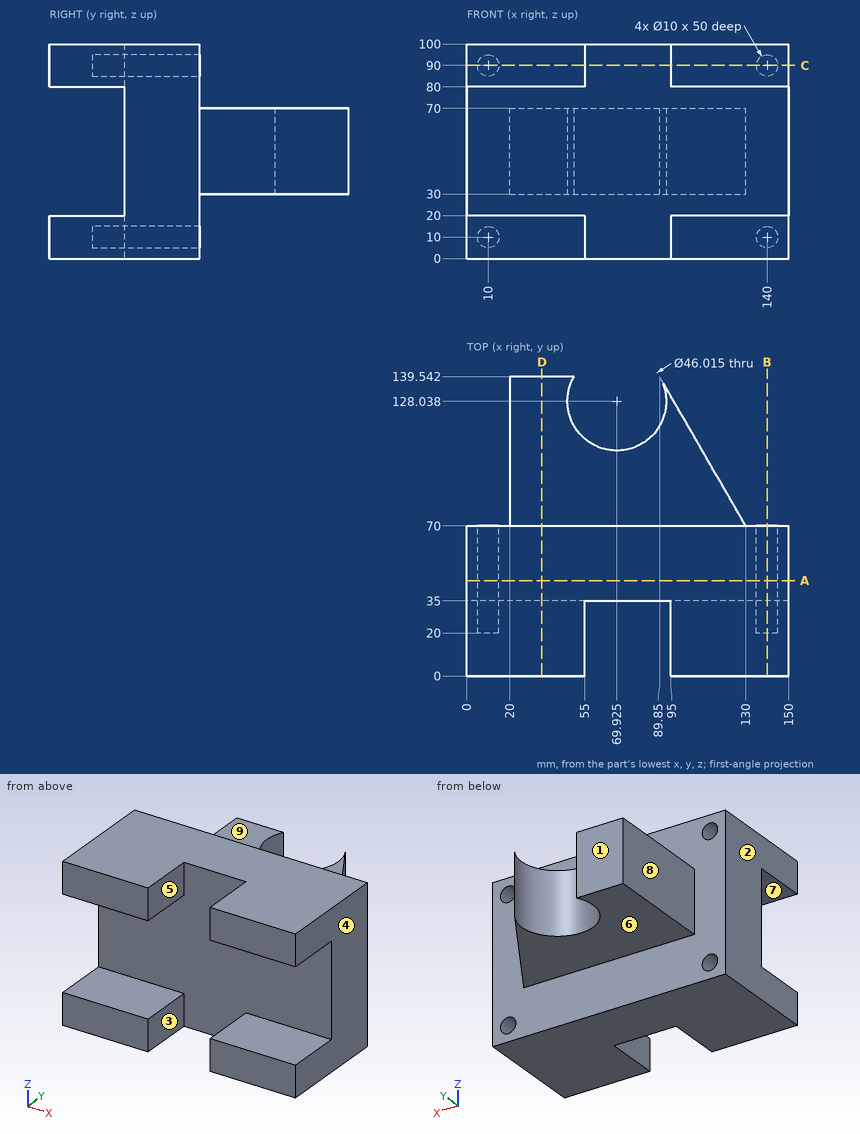
Geometry: see drawing. Coordinates: mm, zero at the bounding-box minimum. A direction names the side the tool comes from. Give positions to 0.01 mm unless a question says otherwise; leave off trailing zeros. Loops run counter-clockwise (first coordinate to the right, second up) from the corner with the lowest first, then second, coordinate; pieces in that order, holes last. Notation, with made-up numbers: (-21.5, 83.25) -> (22.5, 83.25) arc R17 cw to (22.5, 109.25) -> close; hole circle Ø1 at (19.25, 49). An arc over 180 degrees is marked (long way). Use CSV: the item, a comma, the result in double quotes.
(1) Cut plane D-D (x = 35). Output: boundary loops of the cut face in (y, z), plus the area to 3 significant figures.
From the geometry:
outline,"(0, 0) -> (70, 0) -> (70, 30) -> (139.54, 30) -> (139.54, 70) -> (70, 70) -> (70, 100) -> (0, 100) -> (0, 80) -> (35, 80) -> (35, 20) -> (0, 20) -> close"
area,"7,680 mm^2"
(2) Cut plane B-B (x = 140). Output: boundary loops of the cut face in (y, z).
From the geometry:
outline,"(0, 0) -> (70, 0) -> (70, 5) -> (20, 5) -> (20, 15) -> (70, 15) -> (70, 85) -> (20, 85) -> (20, 95) -> (70, 95) -> (70, 100) -> (0, 100) -> (0, 80) -> (35, 80) -> (35, 20) -> (0, 20) -> close"
(3) Cut plane C-C (z = 90). Output: boundary loops of the cut face in (x, y).
From the geometry:
outline,"(0, 0) -> (55, 0) -> (55, 35) -> (95, 35) -> (95, 0) -> (150, 0) -> (150, 70) -> (145, 70) -> (145, 20) -> (135, 20) -> (135, 70) -> (15, 70) -> (15, 20) -> (5, 20) -> (5, 70) -> (0, 70) -> close"
(4) Access query for the marked faces 5, 6, 7, 8 and 9. Directions: +Z, -Z, +X, -X, +Y, -Y. A direction counts if a zero-diameter tool reaches every point of the face in a straight line with its end or side. Return the directions, or none.
From the geometry:
face 5,"+Z, -Z, -Y"
face 6,"-Z, +X, -X, +Y"
face 7,"+X, -X, -Y"
face 8,"+Z, -Z, -X, +Y"
face 9,"+Z, +X, -X, +Y"
(5) Cut plane A-A (y = 44.5). Output: boundary loops of the cut face in (x, z), plus the area to 3 significant figures.
From the geometry:
outline,"(0, 0) -> (150, 0) -> (150, 100) -> (0, 100) -> close; hole circle Ø10 at (10, 10); hole circle Ø10 at (10, 90); hole circle Ø10 at (140, 10); hole circle Ø10 at (140, 90)"
area,"14,700 mm^2"
(6) Ray query, line 1 along Z through (x, y) = (140, 52); line 2 along X through (y, z) = (53, 90); line 3 along Z through (x, y) = (140, 32). Return the intervals inside material, ascending. Write a range as [from, to].
From the geometry:
line 1,"[0, 5], [15, 85], [95, 100]"
line 2,"[0, 5], [15, 135], [145, 150]"
line 3,"[0, 5], [15, 20], [80, 85], [95, 100]"
(7) Pull-direction query (X, two-part tool) for the marked faces 1, 2, 3 and 4; classes: released by +X, released by -X, zero draft, split by the parting line, or undercut.
From the geometry:
face 1,"zero draft"
face 2,"released by -X"
face 3,"undercut"
face 4,"released by +X"
(8) First-contact query: P1, Ø3, axis at x = 139, z = 8.5, coming from the +Y side; P2, Ø2, axis at x = 55, z = 49.5, coming from the +Y side; P3, Ø2, axis at x = 45.5, y = 72, coming from the -Z side; P4, Ø5, axis at x = 105, y = 119.5, coming from the -Z side. Flat tips, straight axial feed; report the tip coordinate or a pass-through.
From the geometry:
P1,"y = 20"
P2,"y = 111.43"
P3,"z = 30"
P4,"through"
